The listing builds one solid part. Answer for the finished solid, in the listing's coordinates (mm). A direction names the side the tool comes from. Coordinates: 2 decimals unless noted, no trailing zeros. Order: outer loops, then holes, each group sorted by start corner. A loop starts at its lowest first (then second) coordinate and runs counter-clockwise, first axis right, second up. Notation, with made-up numbers: (44, 85) - (85, 85) arc R21 cw to (85, 105) - close; hole circle Ø1 at (1.25, 4.25). An arc over 180 degrees is marked (long way). Use a Markdown table: item, result. Add a question column.
Item 1: The part is cut by section D-D, the plane x = 9.5. Give the vertices of the cut face in (y, z), then the cut area to 3 significant figures.
Item 2: Find the intervals of material crossed by line 1 along Y through (x, z) = (81.5, 0); line 2 along Z through (x, y) = (79.75, 0); line 3 along X through (y, z) = (13, -12), in increasing order.
Item 3: For faces 1 (the flat face through (39, 15, -5)), 2 (the cylindrical face through (81, -4, 0)), 3 (the flat face through (39, 5, -15)), 4 (the flat face through (39, -15, -5)), determine the directions among +Z, -Z, +X, -X, +Y, -Y from which every point of the face is accessible in a straight line to the end or side of a thin tool.
Item 4: The part is cut by section A-A, the plane y = 17.5. Give the vertices of the cut face in (x, z).
Item 5: Flat-ended cylindrical pins translate along their axes: P1, Ø4, axis at x = 30, z = 9, coming from the +Y side (3 decimals); P2, Ø3, axis at x = 48.5, y = 14.5, coming from the +Z side; P3, Ø1, axis at x = 29, z = -2, coming from the -Y side. Find the tip coordinate at first contact, or state that the pin passes through.
Item 6: The part is cut by section C-C, the plane y = 0. Give the vertices of the cut face in (x, z), then the cut area to 3 significant figures.
Item 7: The part is cut by section B-B, the plane z = 15.5. Give the vertices of the cut face in (x, y), then the cut area to 3 significant figures.
from build123d import *

# Parameters (mm, degrees)
EXTRUDED_CONNECTOR_DEPTH = 90
KEY_CUT_DEPTH            = 18
CUT_EXTRUDE2_DEPTH       = 10


with BuildPart() as part:
    # Sketch1 → Extruded Connector (new body)
    with BuildSketch(Plane(origin=(0, 0, 0), x_dir=(0, 0, -1), z_dir=(1, 0, 0))):
        with BuildLine():
            ThreePointArc((-19.364916731, -5), (-14.142135624, -14.142135624), (-5, -19.364916731))
            Line((-5, -19.364916731), (-5, -9.964916731))
            Line((-5, -9.964916731), (5, -9.964916731))
            Line((5, -9.964916731), (5, -19.364916731))
            ThreePointArc((5, -19.364916731), (14.142135624, -14.142135624), (19.364916731, -5))
            Line((19.364916731, -5), (9.964916731, -5))
            Line((9.964916731, -5), (9.964916731, 5))
            Line((9.964916731, 5), (19.364916731, 5))
            ThreePointArc((19.364916731, 5), (14.142135624, 14.142135624), (5, 19.364916731))
            Line((5, 19.364916731), (5, 9.964916731))
            Line((5, 9.964916731), (-5, 9.964916731))
            Line((-5, 9.964916731), (-5, 19.364916731))
            ThreePointArc((-5, 19.364916731), (-14.142135624, 14.142135624), (-19.364916731, 5))
            Line((-19.364916731, 5), (-9.964916731, 5))
            Line((-9.964916731, 5), (-9.964916731, -5))
            Line((-9.964916731, -5), (-19.364916731, -5))
        make_face()
    extrude(amount=EXTRUDED_CONNECTOR_DEPTH)

    # Sketch10 → Key Cut (cut)
    with BuildSketch(Plane(origin=(90, 0, 0), x_dir=(0, 0, -1), z_dir=(1, 0, 0))):
        with BuildLine():
            Line((-2.754995463, 2.9), (2.754995463, 2.9))
            ThreePointArc((2.754995463, 2.9), (0, -4), (-2.754995463, 2.9))
        make_face()
    extrude(amount=-KEY_CUT_DEPTH, mode=Mode.SUBTRACT)

    # Sketch11 → Cut-Extrude2 (cut)
    with BuildSketch(Plane(origin=(90, 0, 0), x_dir=(0, 0, -1), z_dir=(1, 0, 0))):
        with BuildLine():
            Line((-9.964916731, 9.964916731), (-9.964916731, 5))
            Line((-9.964916731, 5), (-19.364916731, 5))
            ThreePointArc((-19.364916731, 5), (-14.142135624, 14.142135624), (-5, 19.364916731))
            Line((-5, 19.364916731), (-5, 9.964916731))
            Line((-5, 9.964916731), (-9.964916731, 9.964916731))
        make_face()
        with BuildLine():
            Line((9.964916731, 9.964916731), (5, 9.964916731))
            Line((5, 9.964916731), (5, 19.364916731))
            ThreePointArc((5, 19.364916731), (14.142135624, 14.142135624), (19.364916731, 5))
            Line((19.364916731, 5), (9.964916731, 5))
            Line((9.964916731, 5), (9.964916731, 9.964916731))
        make_face()
        with BuildLine():
            Line((9.964916731, -9.964916731), (9.964916731, -5))
            Line((9.964916731, -5), (19.364916731, -5))
            ThreePointArc((19.364916731, -5), (14.142135624, -14.142135624), (5, -19.364916731))
            Line((5, -19.364916731), (5, -9.964916731))
            Line((5, -9.964916731), (9.964916731, -9.964916731))
        make_face()
        with BuildLine():
            Line((-9.964916731, -9.964916731), (-5, -9.964916731))
            Line((-5, -9.964916731), (-5, -19.364916731))
            ThreePointArc((-5, -19.364916731), (-14.142135624, -14.142135624), (-19.364916731, -5))
            Line((-19.364916731, -5), (-9.964916731, -5))
            Line((-9.964916731, -5), (-9.964916731, -9.964916731))
        make_face()
    extrude(amount=-CUT_EXTRUDE2_DEPTH, mode=Mode.SUBTRACT)


solid = part.part
Solution:
| question | item | result |
|---|---|---|
| 1 | outline | (-19.36, -5) arc R20 ccw to (-5, -19.36) - (-5, -9.96) - (5, -9.96) - (5, -19.36) arc R20 ccw to (19.36, -5) - (9.96, -5) - (9.96, 5) - (19.36, 5) arc R20 ccw to (5, 19.36) - (5, 9.96) - (-5, 9.96) - (-5, 19.36) arc R20 ccw to (-19.36, 5) - (-9.96, 5) - (-9.96, -5) - close |
| 1 | area | 864 mm2 |
| 2 | line 1 | y = -9.96 to -4, 2.9 to 9.96 |
| 2 | line 2 | z = -9.96 to -4, 4 to 9.96 |
| 2 | line 3 | x = 0 to 80 |
| 3 | face 1 | +X, -X, +Y |
| 3 | face 2 | +X |
| 3 | face 3 | -Z, +X, -X |
| 3 | face 4 | +X, -X, -Y |
| 4 | outline | (0, -9.68) - (80, -9.68) - (80, -5) - (0, -5) - close; (0, 5) - (80, 5) - (80, 9.68) - (0, 9.68) - close |
| 5 | P1 | stops at y = 18.735 |
| 5 | P2 | stops at z = 15.2 |
| 5 | P3 | stops at y = -9.96 |
| 6 | outline | (0, -9.96) - (90, -9.96) - (90, -4) - (72, -4) - (72, 4) - (90, 4) - (90, 9.96) - (0, 9.96) - close |
| 6 | area | 1,650 mm2 |
| 7 | outline | (0, -12.64) - (80, -12.64) - (80, -5) - (0, -5) - close; (0, 5) - (80, 5) - (80, 12.64) - (0, 12.64) - close |
| 7 | area | 1,220 mm2 |
